Answer from the drawing. Dimensions are ordinates in mm from the lowest x, y and z of the part. Round coordinates to 2 decimals unless told otherwise and drop trailing zeros. Loops run counter-clockwise (first coordinate to the right, second up) from the corner with the lowest first, then second, coordinate; pieces in that order, holes last. Notation, with made-up numbers: (-5, 47.25) - (52, 47.25) arc R32 cw to (52, 76.25) - close; hole circle Ø5 at (52, 23). An arc over 180 degrees is marked (long way). Answer as CSV lines item,"result". Start each with the question number.
Q1. Section D-D on z = 63 is taken. Write down the section's boundary in (x, y) (1 decimal).
Q2. Section B-B on x = 22 is taken. Write down the section's boundary in (y, z) (1 decimal), then the cut area to 3 significant figures.
Q3. Section C-C on z = 54 is taken. Write down the section's boundary in (x, y) (1 decimal), then the cut area to 3 significant figures.
Q4. Straight lines are drawn through the part: L1, parallel to X at y = 1.35, z = 51 (1 decimal); L2, parallel to Y at x = 13, z = 33; L3, parallel to X at y = 2.5, z = 48 (1 decimal). For each, find the intervals that lie inside material, in ascending order. Write a range as [from, to].
Q5. Each of these flat-tipped pins is pushed along its axis until it touches: pin 1 Ø12 at (x, z) = (66.5, 51.5) entering from -Y; pin 2 Ø1 at (x, y) = (46, 1.5) entering from -Z; pin 3 Ø1.5 at (x, y) = (37, 1.5) entering from -Z. Where does it stop, or does it pass through?
Q6. The mould has two halves that part along Z. Classify the marked faces 1 and 2: +Z half, -Z half, draft (parallel to the pull), parting line (faces both ways), or undercut.
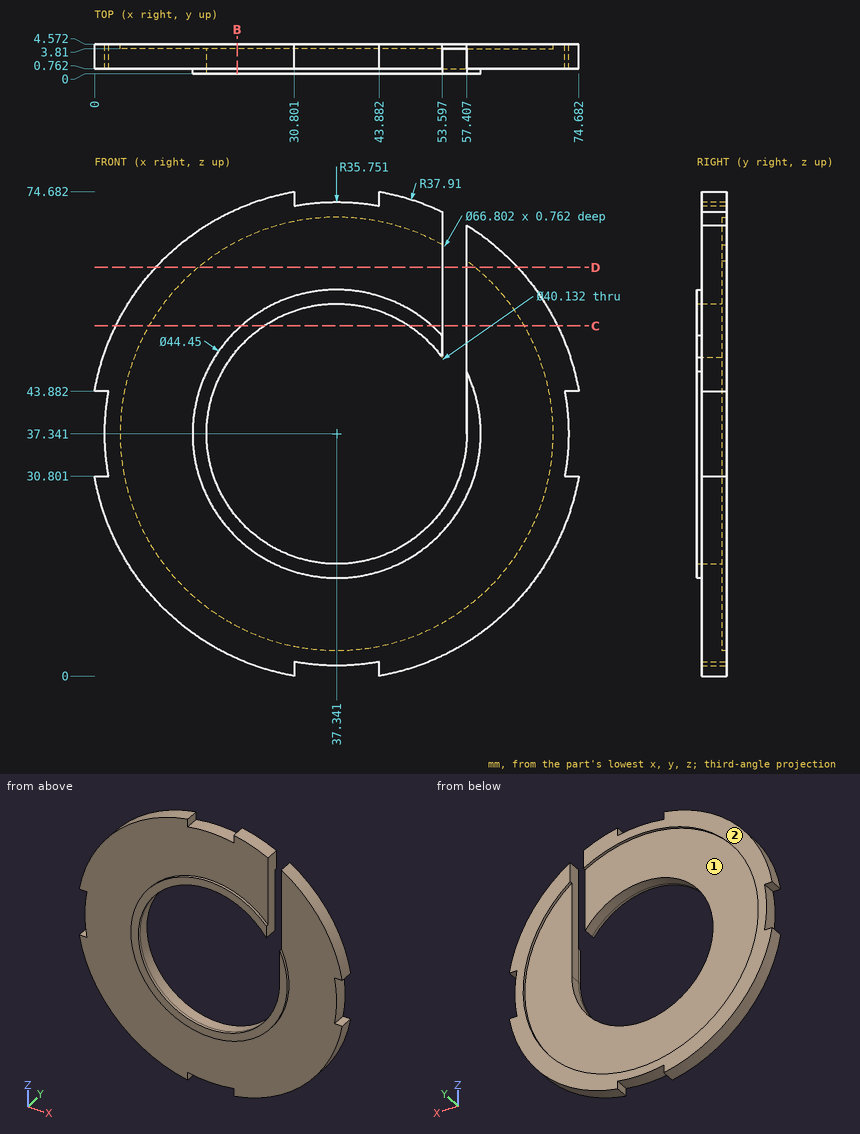
Findings:
1,outline,"(9.4, 0.8) - (53.6, 0.8) - (53.6, 3.8) - (16, 3.8) - (16, 4.6) - (9.4, 4.6) - close; (57.4, 0.8) - (65.2, 0.8) - (65.2, 4.6) - (58.7, 4.6) - (58.7, 3.8) - (57.4, 3.8) - close"
2,outline,"(0, 21.3) - (0.8, 21.3) - (0.8, 2.7) - (4.6, 2.7) - (4.6, 7.7) - (3.8, 7.7) - (3.8, 24.4) - (0, 24.4) - close; (0, 50.3) - (3.8, 50.3) - (3.8, 67) - (4.6, 67) - (4.6, 72) - (0.8, 72) - (0.8, 53.4) - (0, 53.4) - close"
2,area,"145 mm^2"
3,outline,"(3.3, 0.8) - (22.6, 0.8) - (22.6, 0) - (26.2, 0) - (26.2, 3.8) - (8.4, 3.8) - (8.4, 4.6) - (3.3, 4.6) - close; (48.5, 0) - (52.1, 0) - (52.1, 0.8) - (53.6, 0.8) - (53.6, 3.8) - (48.5, 3.8) - close; (57.4, 0.8) - (71.4, 0.8) - (71.4, 4.6) - (66.3, 4.6) - (66.3, 3.8) - (57.4, 3.8) - close"
3,area,"141 mm^2"
4,L1,"x = [2, 22.6], [52, 53.6], [57.4, 72.7]"
4,L2,"y = [0.76, 3.81]"
4,L3,"x = [1, 20.3], [57.4, 73.7]"
5,pin 1,"stops at y = 0.76"
5,pin 2,"stops at z = 0.32"
5,pin 3,"stops at z = 1.59"
6,face 1,"undercut"
6,face 2,"draft"
